For this review, use the dimensioned drawing (mm, ordinates from the lowest corner) and the shaded views. Give positions to 0.01 mm unless a question says otherwise; leave off trailing zeros. Write each loop counter-clockwise with the first axis right and the second up, starting at its lowest first coordinate (ties: lowest second). Pieces come first, ordered by that corner, then holes. Notation, with made-up numbers: (15.25, -5) -> (31.25, -5) arc R24 cw to (31.25, 12) -> close; hole circle Ø10 at (43, 23.5). An arc over 180 degrees is marked (long way). Write each question's results on one line, items separated by ' | '. Start each with the question number.
(1) Take a section at B-B (z = 24). State the section outline as (x, y) points, plus the area to 3 significant figures.
(2) Clearance check with a flat-ended pin moving along its axis: pin 1 (3 mm diameter, centred on x = 39.5, y = 4, fed in from -Z). State where the tip first meets the part, or that it passes through.
(3) Take a section at C-C (y = 1.5). State the section outline as (x, z) points, plus the area to 3 significant figures.
(4) Take a section at D-D (y = 6.75). State the section outline as (x, z) points.
(5) To check wall thickness, follow probe 1 along Z at (x, y) = (5, 5); probe 2 along X at (y, z) = (3, 8.5); probe 3 along X at (y, z) = (0.5, 2.75). State the ranges of each line that lie inside material, in increasing order.
(6) Take a section at A-A (x = 14.5). State the section outline as (y, z) points.
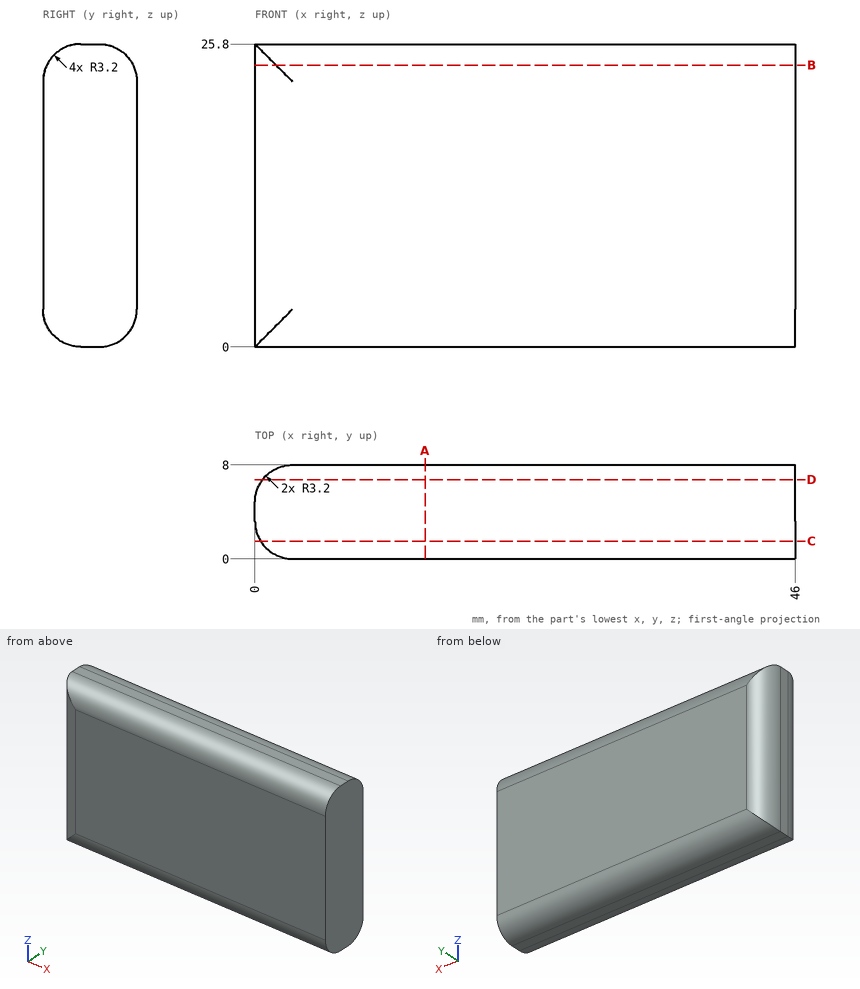
Report:
1) outline: (0, 3.2) arc R3.2 ccw to (1.8, 0.32) -> (46, 0.32) -> (46, 7.68) -> (1.8, 7.68) arc R3.2 ccw to (0, 4.8) -> close | area: 335 mm2
2) pin 1: z = 0
3) outline: (0.49, 0.49) -> (46, 0.49) -> (46, 25.31) -> (0.49, 25.31) -> close | area: 1,130 mm2
4) outline: (0.66, 0.66) -> (46, 0.66) -> (46, 25.14) -> (0.66, 25.14) -> close
5) probe 1: 0.01 to 25.79 | probe 2: 0.01 to 46 | probe 3: 1.48 to 46
6) outline: (0, 3.2) arc R3.2 ccw to (3.2, 0) -> (4.8, 0) arc R3.2 ccw to (8, 3.2) -> (8, 22.6) arc R3.2 ccw to (4.8, 25.8) -> (3.2, 25.8) arc R3.2 ccw to (0, 22.6) -> close
